The listing builds one solid part. Answer for the finished solid, in the listing's coordinates (mm). Face numbers are marked on the shaded views. A direction names the side the tool comes from. Round coordinates to 2 decimals unless told otherwise and drop trailing zeros. Order: outer loops, then holes, each group sorted by start corner. A loop starts at its lowest first (then second) coordinate and runs counter-clockwise, first axis right, second up. Notation, with made-up numbers: (-8.5, -33.75) -> (16.5, -33.75) arc R16 cw to (16.5, -23.75) -> close; hole circle Ø5 at (-9.75, -19.5). An arc over 180 degrees is marked (long way). Answer in a Markdown table with one row per item. Add a question column.
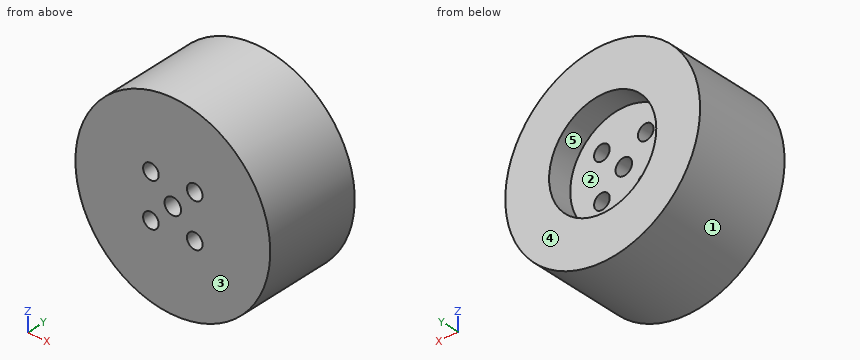
Autodesk Inventor part; units mm, degrees
ref_plane "YZ Plane" through (0, 0, 0) normal (1, 0, 0) x (0, 1, 0)
ref_plane "XZ Plane" through (0, 0, 0) normal (0, 1, 0) x (-1, 0, 0)
ref_plane "XY Plane" through (0, 0, 0) normal (0, 0, 1) x (1, 0, 0)
sketch "Szkic1" plane through (0, 0, 0) normal (0, 1, 0) x (-1, 0, 0)
  circle A0 centre (0, 0) radius 20
  circle A1 centre (0, 0) radius 12.5
  circle A2 centre (0, 0) radius 11
  line L0 (20, 0) -> (-20, 0)
  line L1 (0, 20) -> (0, -20)
  point P0 (4.5, -4.5)
  point P1 (-4.5, -4.5)
  point P2 (4.5, 4.5)
  point P3 (-4.5, 4.5)
  dimension "d0" = 40
  dimension "d1" = 25
  dimension "d2" = 22
  dimension "d3" = 40
  dimension "d6" = 40
  dimension "d35" = 9
  dimension "d36" = 4.5
  dimension "d37" = 4.5
  dimension "d38" = 4.5
extrude "Wyciągnięcie proste1" add sketch "Szkic1" along normal blind 20 contours L0 A1 L1 A0 | A0 L1 A1 L0 | L1 A1 L0 A0 | A0 L0 A1 L1 | L0 A2 L1 A1 | A1 L1 A2 L0 | L1 A2 L0 A1 | A1 L0 A2 L1
extrude "Wyciągnięcie proste2" add sketch "Szkic1" along normal blind 15 contours L0 L1 A2 | A2 L1 L0 | L1 L0 A2 | A2 L0 L1
hole "Otwór2" at (0, 0, 0) direction (0, 1, 0) diameter 3.4 end through all
hole "Hole4" at (-4.5, 0, -4.5) at (4.5, 0, -4.5) at (-4.5, 0, 4.5) at (4.5, 0, 4.5) direction (0, 1, 0) diameter 3.2 depth 30
properties part number "wheel"
1. The part is cut by section D-D (z = -7.5). Give the vertices of the cut face in (x, y), then the cut area to 3 significant figures.
2. Straight lines are drawn through the part: line 1 along X through (y, z) = (11.25, 0); line 2 along X through (y, z) = (8, -4.5). For each, find the intervals that lie inside material, in ascending order.
3. Each of these flat-tipped pins is pushed along its axis until it touches: pin 1 (6.5 mm diameter, centred on x = -4, z = -1.5, fed in from +Y); pin 2 (2 mm diameter, centred on x = 0, z = 0, fed in from +Y); pin 3 (8 mm diameter, centred on x = 9, y = 15.5, fed in from +Z); pin 4 (1.5 mm diameter, centred on x = -10.5, y = 8.5, fed in from +Z). Where does it stop, or does it pass through?
4. The part is cut by section C-C (z = 4.5). Give the vertices of the cut face in (x, y), then the cut area to 3 significant figures.
5. The part is cut by section B-B (y = 10). Give the vertices of the cut face in (x, z), then the cut area to 3 significant figures.
6. For the marked faces 4 and 5, determine the directions among +Z, -Z, +X, -X, +Y, -Y from which every point of the face is accessible in a straight line to the end or side of a thin tool.
7. The mould has two halves that part along Z. Classify the marked faces 1, 2 and 3: released by +Z, released by -Z, zero draft, split by the parting line, or undercut.
8. The part is cut by section A-A (x = 0). Give the vertices of the cut face in (y, z).
Report:
| question | item | result |
|---|---|---|
| 1 | outline | (-18.54, 0) -> (18.54, 0) -> (18.54, 20) -> (8.05, 20) -> (8.05, 15) -> (-8.05, 15) -> (-8.05, 20) -> (-18.54, 20) -> close |
| 1 | area | 661 mm^2 |
| 2 | line 1 | x = -20 to -1.7, 1.7 to 20 |
| 2 | line 2 | x = -19.49 to -6.1, -2.9 to 2.9, 6.1 to 19.49 |
| 3 | pin 1 | stops at y = 15 |
| 3 | pin 2 | passes through |
| 3 | pin 3 | stops at z = 19.36 |
| 3 | pin 4 | stops at z = 17.46 |
| 4 | outline | (-19.49, 0) -> (-6.1, 0) -> (-6.1, 15) -> (-10.04, 15) -> (-10.04, 20) -> (-19.49, 20) -> close; (-2.9, 0) -> (2.9, 0) -> (2.9, 15) -> (-2.9, 15) -> close; (6.1, 0) -> (19.49, 0) -> (19.49, 20) -> (10.04, 20) -> (10.04, 15) -> (6.1, 15) -> close |
| 4 | area | 583 mm^2 |
| 5 | outline | circle Ø40 at (0, 0); hole circle Ø3.2 at (-4.5, -4.5); hole circle Ø3.2 at (-4.5, 4.5); hole circle Ø3.4 at (0, 0); hole circle Ø3.2 at (4.5, -4.5); hole circle Ø3.2 at (4.5, 4.5) |
| 5 | area | 1,220 mm^2 |
| 6 | face 4 | +Z, -Z, +X, -X, +Y |
| 6 | face 5 | +Y |
| 7 | face 1 | split by the parting line |
| 7 | face 2 | undercut |
| 7 | face 3 | zero draft |
| 8 | outline | (0, -20) -> (20, -20) -> (20, -11) -> (15, -11) -> (15, -1.7) -> (0, -1.7) -> close; (0, 1.7) -> (15, 1.7) -> (15, 11) -> (20, 11) -> (20, 20) -> (0, 20) -> close |
